Can you work these out from the model? Positions are in its coordinate system, mm. Face numbers are marked on the shaded views. A direction names the side the tool comes from. Give positions to 0.01 mm unless a question says otherwise; leave off trailing zeros. Loops run counter-clockwise (first coordinate to the right, second up) from the corner with the lowest first, then second, coordinate; pieces in that order, holes last. Notation, with made-up numbers: (-11, 46) - (27, 46) arc R27 cw to (27, 84) - close; hole circle Ø10 at (28, -39.5). An arc over 180 degrees is marked (long way). Answer in a Markdown table with one row per item.
from build123d import *

# Parameters (mm, degrees)
F1_DEPTH = 25.4
F3_DEPTH = 19.05


with BuildPart() as f1:
    # F0 (on Front) → F1 (new body)
    with BuildSketch(Plane.XZ):
        Polygon((0, 12.7), (0, 0), (44.45, 0), (44.45, 6.35), (19.05, 6.35), (19.05, 12.7), align=None)
    extrude(amount=F1_DEPTH)

    # F2 (on face) → F3 (join, through all)
    with BuildSketch(Plane.YZ.offset(19.05)):
        with BuildLine():
            Line((-25.4, 12.7), (0, 12.7))
            ThreePointArc((0, 12.7), (-12.7, 25.4), (-25.4, 12.7))
        make_face()
    extrude(amount=-F3_DEPTH)


solid = f1.part
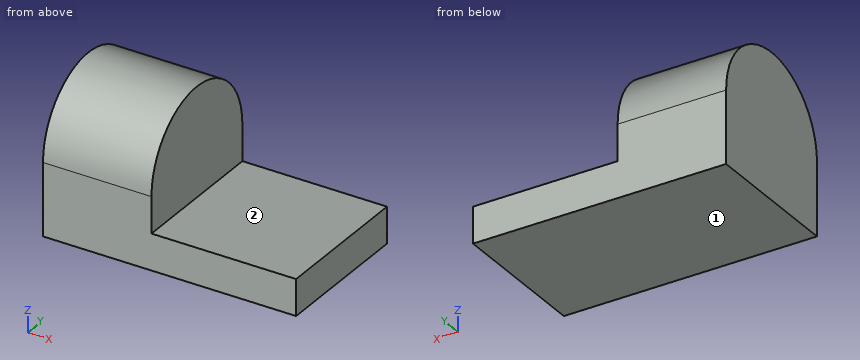
Q1. If I drill on line 1 (X direction, y = -3.5, z = 17); line 2 (Z direction, x = 20.5, y = -9); line 3 (Z direction, x = 5, y = -16.75), over which ranges is the centre line in solid material (lowest first)? Write a range as [from, to].
Checked values:
| item | result |
|---|---|
| line 1 | x = [0, 19.05] |
| line 2 | z = [0, 6.35] |
| line 3 | z = [0, 24.74] |
Q2. Imagine slicing it at D-D, the plane y = -24. Write out the boundary of the cut face in (x, z).
Checked values:
| item | result |
|---|---|
| outline | (0, 0) - (44.45, 0) - (44.45, 6.35) - (19.05, 6.35) - (19.05, 18.5) - (0, 18.5) - close |
Q3. For pin 1 (3 mm diameter, centred on x = 6, y = -10.5, fed in from +Z); pin 2 (5.5 mm diameter, centred on y = -9, z = 13, fed in from +X), each with a flat end and sliding along its axis, tell me the tip position at first contact or that it passes through.
Checked values:
| item | result |
|---|---|
| pin 1 | stops at z = 25.38 |
| pin 2 | stops at x = 19.05 |
Q4. Imagine slicing it at B-B, the plane x = 39. Write out the boundary of the cut face in (y, z), and give its area (3 significant figures).
Checked values:
| item | result |
|---|---|
| outline | (-25.4, 0) - (0, 0) - (0, 6.35) - (-25.4, 6.35) - close |
| area | 161 mm² |
Q5. On a 3-axis mill with a long thin cutter (end or side, diameter ignored), from which of +Z, -Z, +X, -X, +Y, -Y can I reach the whole of each face in a straight line? I mean the marked faces 1 and 2. Say none if no direction works.
Checked values:
| item | result |
|---|---|
| face 1 | -Z, +X, -X, +Y, -Y |
| face 2 | +Z, +X, +Y, -Y |
Q6. Imagine slicing it at A-A, the plane y = -12.7. Write out the boundary of the cut face in (x, z).
Checked values:
| item | result |
|---|---|
| outline | (0, 0) - (44.45, 0) - (44.45, 6.35) - (19.05, 6.35) - (19.05, 25.4) - (0, 25.4) - close |
Q7. Imagine slicing it at C-C, the plane z = 23. Write out the boundary of the cut face in (x, y), and give its area (3 significant figures).
Checked values:
| item | result |
|---|---|
| outline | (0, -20.13) - (19.05, -20.13) - (19.05, -5.27) - (0, -5.27) - close |
| area | 283 mm² |
